```python
from build123d import *

# Parameters (mm, degrees)
PAD_DEPTH       = 4
SKETCH001_R     = 1.45
HOLE_DEPTH      = 4.001
SKETCH002_W     = 7
SKETCH002_H     = 11
POCKET_DEPTH    = 4.001
SKETCH003_R     = 2.1
POCKET001_DEPTH = 4.001
SKETCH004_R     = 1.7
HOLE001_DEPTH   = 4.001
POCKET002_DEPTH = 4.001


with BuildPart() as part:
    # Sketch → Pad (new body)
    with BuildSketch(Plane.XY):
        with BuildLine():
            Line((-25, -32.5), (25, -32.5))
            ThreePointArc((25, -32.5), (27.12132, -31.62132), (28, -29.5))
            Line((28, -29.5), (28, 29.5))
            ThreePointArc((28, 29.5), (27.12132, 31.62132), (25, 32.5))
            Line((25, 32.5), (-25, 32.5))
            ThreePointArc((-25, 32.5), (-27.12132, 31.62132), (-28, 29.5))
            Line((-28, 29.5), (-28, -29.5))
            ThreePointArc((-28, -29.5), (-27.12132, -31.62132), (-25, -32.5))
        make_face()
    extrude(amount=PAD_DEPTH)

    # Sketch001 (on Face10 of Pad) → Hole (cut, through all)
    with BuildSketch(Plane.XY.offset(4)):
        with Locations((24.5, -29)):
            Circle(SKETCH001_R)
        with Locations((-24.5, -29)):
            Circle(SKETCH001_R)
        with Locations((-24.5, 29)):
            Circle(SKETCH001_R)
        with Locations((24.5, 29)):
            Circle(SKETCH001_R)
    extrude(amount=-HOLE_DEPTH, mode=Mode.SUBTRACT)

    # Sketch002 (on Face5 of Hole) → Pocket (cut, through all)
    with BuildSketch(Plane.XY.offset(4)):
        with Locations((-24.5, -20)):
            Rectangle(SKETCH002_W, SKETCH002_H)
    extrude(amount=-POCKET_DEPTH, mode=Mode.SUBTRACT)

    # Sketch003 (on Face5 of Pocket) → Pocket001 (cut, through all)
    with BuildSketch(Plane.XY.offset(4)):
        with Locations((7.5, 25)):
            Circle(SKETCH003_R)
        with Locations((-20.5, 7.5)):
            Circle(SKETCH003_R)
    extrude(amount=-POCKET001_DEPTH, mode=Mode.SUBTRACT)

    # Sketch004 (on Face5 of Pocket001) → Hole001 (cut, through all)
    with BuildSketch(Plane.XY.offset(4)):
        with Locations((-20.5, -7.5)):
            Circle(SKETCH004_R)
        with Locations((-7.5, 25)):
            Circle(SKETCH004_R)
    extrude(amount=-HOLE001_DEPTH, mode=Mode.SUBTRACT)

    # Sketch005 (on Face5 of Hole001) → Pocket002 (cut, through all)
    with BuildSketch(Plane.XY.offset(4)):
        with BuildLine():
            Line((-9.5, 17.5), (9.5, 17.5))
            ThreePointArc((13, 14), (11.974874, 16.474874), (9.5, 17.5))
            Line((13, 14), (13, -14))
            ThreePointArc((9.5, -17.5), (11.974874, -16.474874), (13, -14))
            Line((9.5, -17.5), (-9.5, -17.5))
            ThreePointArc((-13, -14), (-11.974874, -16.474874), (-9.5, -17.5))
            Line((-13, -14), (-13, 14))
            ThreePointArc((-9.5, 17.5), (-11.974874, 16.474874), (-13, 14))
        make_face()
    extrude(amount=-POCKET002_DEPTH, mode=Mode.SUBTRACT)


solid = part.part
```
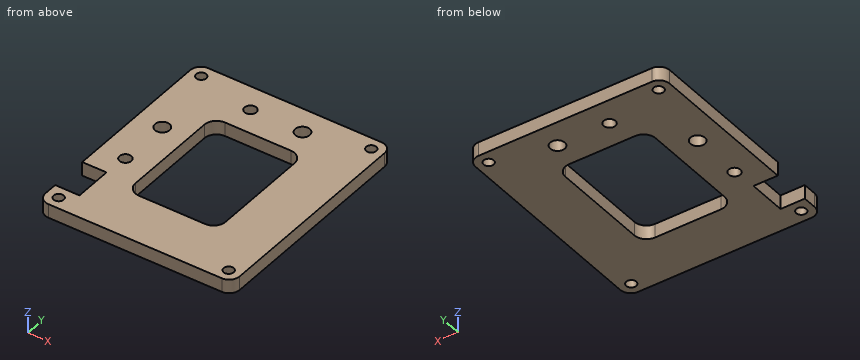
Part model, mm, in its own coordinate system. Round coordinates to 2 decimals unless told otherwise and drop trailing zeros. Loops run counter-clockwise (first coordinate to the right, second up) from the corner with the lowest first, then second, coordinate; pieces in that order, holes last.
1. Flat gauge pin, fed straight in: pin 1 (1.2 mm diameter, centred on y = -22.5, z = 1.5, fed in from -X). Where does the tip first touch, or does it go through?
Solutions:
pin 1: stops at x = -21
2. Slice it at B-B (x = 3). Give the cut face in (y, z), and give its area (3 significant figures).
Solutions:
outline: (-32.5, 0) - (-17.5, 0) - (-17.5, 4) - (-32.5, 4) - close; (17.5, 0) - (32.5, 0) - (32.5, 4) - (17.5, 4) - close
area: 120 mm2
3. Drill centre lines: line 1 along Y through (x, z) = (24.5, 2.45); line 2 along Y through (x, z) = (-7.5, 1.9); line 3 along Y through (x, z) = (3.5, 1.5). Where is each one in solid material? Low to high.
Solutions:
line 1: y = -32.5 to -30.45, -27.55 to 27.55, 30.45 to 32.5
line 2: y = -32.5 to -17.5, 17.5 to 23.3, 26.7 to 32.5
line 3: y = -32.5 to -17.5, 17.5 to 32.5
4. Slice it at D-D (y = 13). Give the cut face in (x, z).
Solutions:
outline: (-28, 0) - (-13, 0) - (-13, 4) - (-28, 4) - close; (13, 0) - (28, 0) - (28, 4) - (13, 4) - close
5. Slice it at A-A (y = -7.5). Give the cut face in (x, z).
Solutions:
outline: (-28, 0) - (-22.2, 0) - (-22.2, 4) - (-28, 4) - close; (-18.8, 0) - (-13, 0) - (-13, 4) - (-18.8, 4) - close; (13, 0) - (28, 0) - (28, 4) - (13, 4) - close
6. Slice it at C-C (z = 2.2). Count the separate pieces of the cut face and the enclosed holes in it, and give its area (3 significant figures).
Solutions:
separate pieces: 1
enclosed holes: 9
area: 2,580 mm2
